Geometry: final body of the model. Coordinates: model frame, mm. Round coordinates to 2 decimals unless told otherwise and drop trailing zeros. Loops run counter-clockwise (first coordinate to the right, second up) from the corner with the lowest first, then second, coordinate; pieces in that order, holes last. Notation, with made-up numbers: (42, 46.25) -> (59, 46.25) arc R29 cw to (59, 77.25) -> close; hole circle Ø3 at (-32.5, 24.5). An arc over 180 degrees is marked (long way). Answer in a Markdown table with one row per item.
```python
from build123d import *

# Parameters (mm, degrees)
SKETCH1_R                = 2.4638
BOSS_EXTRUDE1_DEPTH      = 3.175
SKETCH2_R                = 1.9431
SKETCH2_W                = 16.51
SKETCH2_H                = 13.843
CUT_EXTRUDE1_DEPTH       = 159.781746826
SKETCH5_R                = 3.175
SKETCH5_R_2              = 2.159
SKETCH5_R_3              = 1.4478
CUT_EXTRUDE2_DEPTH       = 159.781746826
SKETCH6_R                = 2.159
CUT_EXTRUDE3_DEPTH       = 159.781746826
SKETCH5_3_R              = 1.45415
CUT_EXTRUDE4_DEPTH       = 159.781746826
SKETCH5_4_R              = 1.5875
SKETCH5_4_R_2            = 4.7625
CUT_EXTRUDE5_DEPTH       = 159.781746826
SKETCH5_5_R              = 1.5875
CUT_EXTRUDE6_DEPTH       = 2.54
CUT_EXTRUDE7_START       = -3.175
CUT_EXTRUDE7_OUTLINE_R   = 1.5875
CUT_EXTRUDE7_DEPTH       = 0.635
CUT_EXTRUDE8_DEPTH       = 7.62
CUT_EXTRUDE8_DEPTH_BACK  = 2.54
SKETCH5_7_R              = 1.5875
SKETCH5_7_W              = 9.525
SKETCH5_7_H              = 19.05
SKETCH5_9_R              = 1.5875
CUT_EXTRUDE9_DEPTH       = 159.781746826
CUT_EXTRUDE17_DEPTH      = 159.781746826
CUT_EXTRUDE17_DEPTH_BACK = 159.781746826
SKETCH5_15_W             = 9.525
SKETCH5_15_H             = 19.05
FILLET1_R                = 2.54
FILLET2_R                = 2.54
FILLET3_R                = 2.54
FILLET4_R                = 2.54
SKETCH9_R                = 1.55
SKETCH9_R_2              = 2
CUT_EXTRUDE18_DEPTH      = 159.781746826
SKETCH3_R                = 1.5875
CUT_EXTRUDE19_DEPTH      = 976.122


# Read off the part's stored shape, not the designer's step: Cut-Extrude7
with BuildPart() as part:
    # Sketch1 → Boss-Extrude1 (new body)
    with BuildSketch(Plane.XY):
        Polygon((-111.686526805, -95.25), (-127, -83.918625912), (-127, 83.918625912), (-111.686526805, 95.25), (111.686526805, 95.25), (127, 83.918625912), (127, -83.918625912), (111.686526805, -95.25), align=None)
        with Locations((-95.147512794, 56.885632681)):
            Circle(SKETCH1_R, mode=Mode.SUBTRACT)
        with Locations((-110.256011578, 77.303596941)):
            Circle(SKETCH1_R, mode=Mode.SUBTRACT)
        with Locations(Location((110.256011578, 77.303596941, 0), (0, 0, 180))):
            Circle(SKETCH1_R, mode=Mode.SUBTRACT)
        with Locations(Location((95.147512794, 56.885632681, 0), (0, 0, 180))):
            Circle(SKETCH1_R, mode=Mode.SUBTRACT)
        with Locations(Location((-110.256011578, -77.303596941, 0), (0, 0, 180))):
            Circle(SKETCH1_R, mode=Mode.SUBTRACT)
        with Locations(Location((-95.147512794, -56.885632681, 0), (0, 0, 180))):
            Circle(SKETCH1_R, mode=Mode.SUBTRACT)
        with Locations((110.256011578, -77.303596941)):
            Circle(SKETCH1_R, mode=Mode.SUBTRACT)
        with Locations((95.147512794, -56.885632681)):
            Circle(SKETCH1_R, mode=Mode.SUBTRACT)
    extrude(amount=BOSS_EXTRUDE1_DEPTH)

    # Sketch2 → Cut-Extrude1 (cut, through all)
    with BuildSketch(Plane.XY.offset(3.175)):
        with Locations((68.326, -56.00521613)):
            Circle(SKETCH2_R)
        with Locations((45.974, -56.00521613)):
            Circle(SKETCH2_R)
        with Locations((57.15, -56.00521613)):
            Rectangle(SKETCH2_W, SKETCH2_H)
    extrude(amount=-CUT_EXTRUDE1_DEPTH, mode=Mode.SUBTRACT)

    # Sketch5 → Cut-Extrude2 (cut, through all)
    with BuildSketch(Plane(origin=(0, 0, 0), x_dir=(-1, 0, 0), z_dir=(0, 0, -1))):
        with Locations((82.55, 57.21604)):
            Circle(SKETCH5_R)
        with Locations((61.9506, 48.13554)):
            Circle(SKETCH5_R_2)
        with Locations((103.9495, 48.13554)):
            Circle(SKETCH5_R_2)
        with Locations((61.9506, -48.13554)):
            Circle(SKETCH5_R_2)
        with Locations((103.9495, -48.13554)):
            Circle(SKETCH5_R_2)
        with Locations((56.479426463, 15.03413)):
            Circle(SKETCH5_R_3)
        with Locations((56.479426463, -15.03413)):
            Circle(SKETCH5_R_3)
        with Locations((86.197426463, -15.03413)):
            Circle(SKETCH5_R_3)
        with Locations((86.197426463, 15.03413)):
            Circle(SKETCH5_R_3)
        with BuildLine():
            Line((-25.4, 25.4), (-25.4, -25.4))
            ThreePointArc((-25.4, -25.4), (-28.575, -28.575), (-31.75, -25.4))
            Line((-31.75, -25.4), (-31.75, 25.4))
            ThreePointArc((-31.75, 25.4), (-28.575, 28.575), (-25.4, 25.4))
        make_face()
        with BuildLine():
            Line((25.4, 25.4), (25.4, -25.4))
            ThreePointArc((25.4, -25.4), (28.575, -28.575), (31.75, -25.4))
            Line((31.75, -25.4), (31.75, 25.4))
            ThreePointArc((31.75, 25.4), (28.575, 28.575), (25.4, 25.4))
        make_face()
    extrude(amount=-CUT_EXTRUDE2_DEPTH, mode=Mode.SUBTRACT)

    # Sketch6 → Cut-Extrude3 (cut, through all)
    with BuildSketch(Plane(origin=(0, 0, 0), x_dir=(-1, 0, 0), z_dir=(0, 0, -1))):
        with Locations((-76.2, -85.725)):
            Circle(SKETCH6_R)
        with Locations((-25.4, -85.725)):
            Circle(SKETCH6_R)
        with Locations((25.4, -85.725)):
            Circle(SKETCH6_R)
        with Locations((76.2, -85.725)):
            Circle(SKETCH6_R)
        with Locations(Location((76.2, 85.725, 0), (0, 0, 180))):
            Circle(SKETCH6_R)
        with Locations(Location((25.4, 85.725, 0), (0, 0, 180))):
            Circle(SKETCH6_R)
        with Locations(Location((-25.4, 85.725, 0), (0, 0, 180))):
            Circle(SKETCH6_R)
        with Locations(Location((-76.2, 85.725, 0), (0, 0, 180))):
            Circle(SKETCH6_R)
        with Locations((117.475, -25.4)):
            Circle(SKETCH6_R)
        with Locations(Location((117.475, 25.4, 0), (0, 0, 180))):
            Circle(SKETCH6_R)
        with Locations((-117.475, 25.4)):
            Circle(SKETCH6_R)
        with Locations(Location((-117.475, -25.4, 0), (0, 0, 180))):
            Circle(SKETCH6_R)
    extrude(amount=-CUT_EXTRUDE3_DEPTH, mode=Mode.SUBTRACT)

    # Sketch5_3 → Cut-Extrude4 (cut, through all)
    with BuildSketch(Plane(origin=(0, 0, 0), x_dir=(-1, 0, 0), z_dir=(0, 0, -1))):
        with Locations((-42.5, 17.2)):
            Circle(SKETCH5_3_R)
        with Locations(Location((-42.5, -17.2, 0), (0, 0, 180))):
            Circle(SKETCH5_3_R)
        with Locations((42.5, -17.2)):
            Circle(SKETCH5_3_R)
        with Locations(Location((42.5, 17.2, 0), (0, 0, 180))):
            Circle(SKETCH5_3_R)
    extrude(amount=-CUT_EXTRUDE4_DEPTH, mode=Mode.SUBTRACT)

    # Sketch5_4 → Cut-Extrude5 (cut, through all)
    with BuildSketch(Plane(origin=(0, 0, 0), x_dir=(-1, 0, 0), z_dir=(0, 0, -1))):
        with Locations(Location((61.544630637, -54.61, 0), (0, 0, 180))):
            Circle(SKETCH5_4_R)
        with Locations((61.544630637, -67.31)):
            Circle(SKETCH5_4_R)
        with Locations((-60.325, -85.725)):
            Circle(SKETCH5_4_R_2)
        with Locations((61.544630637, 54.61)):
            Circle(SKETCH5_4_R)
        with Locations(Location((40.055369363, -67.31, 0), (0, 0, 180))):
            Circle(SKETCH5_4_R_2)
        with Locations(Location((61.544630637, 67.31, 0), (0, 0, 180))):
            Circle(SKETCH5_4_R)
        with Locations((40.055369363, 67.31)):
            Circle(SKETCH5_4_R_2)
    extrude(amount=-CUT_EXTRUDE5_DEPTH, mode=Mode.SUBTRACT)

    # Sketch5_5 → Cut-Extrude6 (cut)
    with BuildSketch(Plane(origin=(0, 0, 0), x_dir=(-1, 0, 0), z_dir=(0, 0, -1))):
        with Locations(Location((38.886108088, 54.61, 0), (0, 0, 180))):
            Circle(SKETCH5_5_R)
    extrude(amount=-CUT_EXTRUDE6_DEPTH, mode=Mode.SUBTRACT)

    # Cut-Extrude7 outline → Cut-Extrude7 (cut)
    with BuildSketch(Plane(origin=(0, 0, 0), x_dir=(-1, 0, 0), z_dir=(0, 0, -1)).offset(CUT_EXTRUDE7_START)):
        with Locations((38.886108088, 54.61)):
            Circle(CUT_EXTRUDE7_OUTLINE_R)
    extrude(amount=CUT_EXTRUDE7_DEPTH, mode=Mode.SUBTRACT)

    # Sketch5_7 → Cut-Extrude8 (cut, two sides: drawn at the far end of the back side and taken through both)
    with BuildSketch(Plane(origin=(0, 0, 0), x_dir=(-1, 0, 0), z_dir=(0, 0, -1)).offset(-CUT_EXTRUDE8_DEPTH_BACK)):
        with Locations(Location((40.055369363, -54.61, 0), (0, 0, 180))):
            Circle(SKETCH5_7_R)
        with Locations((-50.8, 76.2)):
            Rectangle(SKETCH5_7_W, SKETCH5_7_H)
    extrude(amount=CUT_EXTRUDE8_DEPTH + CUT_EXTRUDE8_DEPTH_BACK, mode=Mode.SUBTRACT)

    # Sketch5_9 → Cut-Extrude9 (cut, through all)
    with BuildSketch(Plane(origin=(0, 0, 0), x_dir=(-1, 0, 0), z_dir=(0, 0, -1))):
        with Locations(Location((40.055369363, -54.61, 0), (0, 0, 180))):
            Circle(SKETCH5_9_R)
    extrude(amount=-CUT_EXTRUDE9_DEPTH, mode=Mode.SUBTRACT)

    # Sketch5_15 → Cut-Extrude17 (cut, two sides: drawn at the far end of the back side and taken through both)
    with BuildSketch(Plane(origin=(0, 0, 0), x_dir=(-1, 0, 0), z_dir=(0, 0, -1)).offset(-CUT_EXTRUDE17_DEPTH_BACK)):
        with Locations((-50.8, 76.2)):
            Rectangle(SKETCH5_15_W, SKETCH5_15_H)
    extrude(amount=CUT_EXTRUDE17_DEPTH + CUT_EXTRUDE17_DEPTH_BACK, mode=Mode.SUBTRACT)

    # Fillet1
    fillet1_edges = [part.edges().sort_by_distance(p)[0] for p in [
        (55.5625, 85.725, 1.5875),
    ]]
    fillet(fillet1_edges, radius=FILLET1_R)

    # Fillet2
    fillet2_edges = [part.edges().sort_by_distance(p)[0] for p in [
        (46.0375, 85.725, 1.5875),
    ]]
    fillet(fillet2_edges, radius=FILLET2_R)

    # Fillet3
    fillet3_edges = [part.edges().sort_by_distance(p)[0] for p in [
        (46.0375, 66.675, 1.5875),
    ]]
    fillet(fillet3_edges, radius=FILLET3_R)

    # Fillet4
    fillet4_edges = [part.edges().sort_by_distance(p)[0] for p in [
        (55.5625, 66.675, 1.5875),
    ]]
    fillet(fillet4_edges, radius=FILLET4_R)

    # Sketch9 → Cut-Extrude18 (cut, through all)
    with BuildSketch(Plane.XY.offset(3.175)):
        with Locations((34.370000094, 30.350000006)):
            Circle(SKETCH9_R)
        with Locations((64.77, 30.350000006)):
            Circle(SKETCH9_R)
        with Locations((64.77, 6.35)):
            Circle(SKETCH9_R)
        with Locations((34.370000094, 6.35)):
            Circle(SKETCH9_R)
        with Locations((68.58, 69.85)):
            Circle(SKETCH9_R_2)
        with Locations((39.58, 69.85)):
            Circle(SKETCH9_R_2)
        with Locations((39.58, 42.35)):
            Circle(SKETCH9_R_2)
        with Locations((68.58, 42.35)):
            Circle(SKETCH9_R_2)
    extrude(amount=-CUT_EXTRUDE18_DEPTH, mode=Mode.SUBTRACT)

    # Sketch3 → Cut-Extrude19 (cut)
    with BuildSketch(Plane.XY.offset(3.175)):
        with Locations((-15.875, -65.560310834)):
            Circle(SKETCH3_R)
        with Locations((15.875, -65.560310834)):
            Circle(SKETCH3_R)
        with Locations((-15.875, -54.130310834)):
            Circle(SKETCH3_R)
        with Locations((15.875, -54.130310834)):
            Circle(SKETCH3_R)
    extrude(amount=-CUT_EXTRUDE19_DEPTH, mode=Mode.SUBTRACT)


solid = part.part
```
Item 1: Draft query along X for faces 1 (the face through (-84.26, 59.89, 1.57)), 2 (the face through (-119.45, 89.505, 1.565)), 3 (the face through (2, 1, 3.175)). Return one class per face: pulls with the +X half, pulls with the -X half, needs draft (parallel to the pull), parting line crosses it, or undercut.
Answer:
| item | result |
|---|---|
| face 1 | undercut |
| face 2 | pulls with the -X half |
| face 3 | needs draft |
Item 2: Cut plane A-A (y = -7.5). Output: boundary loops of the cut face in (x, z) (3 decimals).
Answer:
| item | result |
|---|---|
| outline | (-127, 0) -> (-31.75, 0) -> (-31.75, 3.175) -> (-127, 3.175) -> close; (-25.4, 0) -> (25.4, 0) -> (25.4, 3.175) -> (-25.4, 3.175) -> close; (31.75, 0) -> (127, 0) -> (127, 3.175) -> (31.75, 3.175) -> close |
Item 3: Pin query (flat end, axial travel): pin 1 Ø1.9 at (x, y) = (-61.54, 67.31) entering from +Z. Return the tip coordinate at first contact, or that it passes through.
Answer:
| item | result |
|---|---|
| pin 1 | passes through |
Item 4: Cut plane B-B (z = 0.55). Count the separate pieces of the cut face and the enclosed holes in it, then the cut area to 3 significant figures.
Answer:
| item | result |
|---|---|
| separate pieces | 1 |
| enclosed holes | 60 |
| area | 46,100 mm² |
Item 5: Line query: probe 1 along X at (y, z) = (21, 1.8); probe 2 along X at (y, z) = (80.5, 2); probe 3 along X at (y, z) = (30, 2.45). Output: solid intervals per line, ascending. Write a range as [from, to].
Answer:
| item | result |
|---|---|
| probe 1 | x = [-127, -31.75], [-25.4, 25.4], [31.75, 127] |
| probe 2 | x = [-127, 46.04], [55.56, 127] |
| probe 3 | x = [-127, 32.86], [35.88, 63.26], [66.28, 127] |
